Read the model definition and answer for the solid it produces. Units are mm, in the model's axes. Coordinates: 2 decimals unless noted, no trailing zeros. Order: outer loops, then holes, each group sorted by start corner. A loop starts at its lowest first (then second) coordinate and runs counter-clockwise, first axis right, second up. Notation, with made-up numbers: (15, -11.5) -> (30, -11.5) arc R17 ccw to (30, 10.5) -> close; hole circle Ø3 at (60.25, -36). An arc over 180 degrees is marked (long way). Answer as a JSON object with one key per item and string values. Group by question number.
1) Given pin 1 (0.9 mm diameter, centred on y = -1.5, z = 2, fed in from +X); pin 2 (1.5 mm diameter, centred on y = -20, z = 1, fed in from -X); pin 3 (2 mm diameter, centred on x = -25.5, y = -8.5, fed in from -Z); pin 4 (1.5 mm diameter, centred on x = -1.5, z = 2, fed in from +Y), each flat-ended and moving along its own axis, determine where each tip first touches the part or whether it passes through.
2) Consider L1, parallel to Y at x = -32.5, z = 2; L2, parallel to Y at x = 15.25, z = 1.95; L3, parallel to X at y = 16, z = 0.35. Determine where each line is inside the solid, lowest interval first.
3) Section A-A on x = 15.25 is taken. Determine the outline of the cut face in (y, z).
4) Section D-D on x = -5 is taken. Determine the outline of the cut face in (y, z).
5) Section B-B on x = -40 is taken. Determine the outline of the cut face in (y, z), and give its area (3 significant figures).
6) Section C-C on z = 1.25 is taken. Count the separate pieces of the cut face and the enclosed holes in it, and give its area (3 significant figures).
from build123d import *

# Parameters (mm, degrees)
F0_R     = 1.5
F0_W     = 25
F0_H     = 3
F1_DEPTH = 3


with BuildPart() as f1:
    # F0 (on Top) → F1 (new body)
    with BuildSketch(Plane.XY):
        Polygon((5.826227, 25), (-10, 25), (-15.97664, 30.97664), (-45.976639, 30.97664), (-37, 22), (-37, -22), (-45.976639, -30.97664), (-15.97664, -30.97664), (-10, -25), (5.826227, -25), (12.348584, -30.97664), (30.97664, -30.97664), (30.97664, -19.30114), (23, -11.991897), (23, 11.991897), (30.97664, 19.30114), (30.97664, 30.97664), (12.348584, 30.97664), align=None)
        with Locations((-32.5, -13)):
            Circle(F0_R, mode=Mode.SUBTRACT)
        with Locations((-15.25, -15.25)):
            Circle(F0_R, mode=Mode.SUBTRACT)
        with Locations((0, -20.5)):
            Rectangle(F0_W, F0_H, mode=Mode.SUBTRACT)
        with Locations((18, -22.5)):
            Circle(F0_R, mode=Mode.SUBTRACT)
        with Locations((15.25, -15.25)):
            Circle(F0_R, mode=Mode.SUBTRACT)
        with Locations((-32.5, 13)):
            Circle(F0_R, mode=Mode.SUBTRACT)
        with Locations((-15.25, 15.25)):
            Circle(F0_R, mode=Mode.SUBTRACT)
        with Locations((15.25, 15.25)):
            Circle(F0_R, mode=Mode.SUBTRACT)
        with Locations((0, 20.5)):
            Rectangle(F0_W, F0_H, mode=Mode.SUBTRACT)
        with Locations((18, 22.5)):
            Circle(F0_R, mode=Mode.SUBTRACT)
    extrude(amount=F1_DEPTH)


solid = f1.part
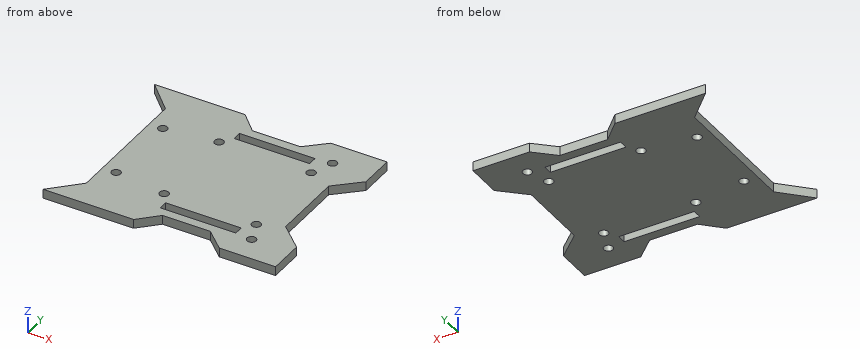
Worked answers:
{
 "1": {"pin 1": "stops at x = 23", "pin 2": "stops at x = -37", "pin 3": "stops at z = 0", "pin 4": "stops at y = 25"},
 "2": {"L1": "y = -30.98 to -14.5, -11.5 to 11.5, 14.5 to 30.98", "L2": "y = -30.98 to -16.75, -13.75 to 13.75, 16.75 to 30.98", "L3": "x = -37 to -16.55, -13.95 to 13.95, 16.55 to 27.37"},
 "3": {"outline": "(-30.98, 0) -> (-16.75, 0) -> (-16.75, 3) -> (-30.98, 3) -> close; (-13.75, 0) -> (13.75, 0) -> (13.75, 3) -> (-13.75, 3) -> close; (16.75, 0) -> (30.98, 0) -> (30.98, 3) -> (16.75, 3) -> close"},
 "4": {"outline": "(-25, 0) -> (-22, 0) -> (-22, 3) -> (-25, 3) -> close; (-19, 0) -> (19, 0) -> (19, 3) -> (-19, 3) -> close; (22, 0) -> (25, 0) -> (25, 3) -> (22, 3) -> close"},
 "5": {"outline": "(-30.98, 0) -> (-25, 0) -> (-25, 3) -> (-30.98, 3) -> close; (25, 0) -> (30.98, 0) -> (30.98, 3) -> (25, 3) -> close", "area": "35.9 mm²"},
 "6": {"separate pieces": "1", "enclosed holes": "10", "area": "3,570 mm²"}
}
